Build history of the part. All positions in model axes, mm. Face numbers are marked on the shaded views. A direction names the side the tool comes from. Give positions to 0.01 mm unless a question says otherwise; leave off trailing zeros. Write each loop counter-clockwise with the first axis right and the second up, starting at its lowest first coordinate (ties: lowest second). Pieces come first, ordered by that corner, then holes. Notation, with made-up numbers: (86, 50) -> (92, 50) arc R25 cw to (92, 87) -> close; hole circle Ø10 at (80.25, 7). An arc over 180 degrees is marked (long way). Put each result on its own line as item: value.
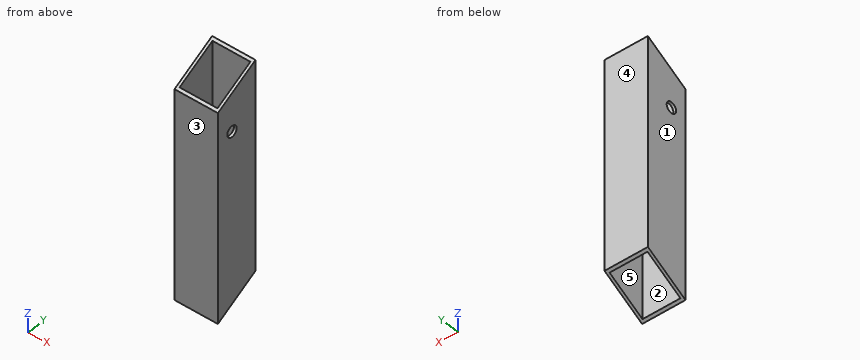
Autodesk Inventor part; units mm, degrees
ref_plane "YZ Plane" through (0, 0, 0) normal (1, 0, 0) x (0, 1, 0)
ref_plane "XZ Plane" through (0, 0, 0) normal (0, 1, 0) x (-1, 0, 0)
ref_plane "XY Plane" through (0, 0, 0) normal (0, 0, 1) x (1, 0, 0)
sketch "Sketch1" plane through (0, 0, 0) normal (0, 0, 1) x (1, 0, 0)
  line L0 (0, 0) -> (25.4, 0)
  line L1 (25.4, 0) -> (25.4, 25.4)
  line L2 (25.4, 25.4) -> (0, 25.4)
  line L3 (0, 25.4) -> (0, 0)
  line L4 (1.5875, 23.8125) -> (23.8125, 23.8125)
  line L5 (23.8125, 23.8125) -> (23.8125, 1.5875)
  line L6 (23.8125, 1.5875) -> (1.5875, 1.5875)
  line L7 (1.5875, 1.5875) -> (1.5875, 23.8125)
  dimension "d0" = 25.4
  dimension "d1" = 25.4
  dimension "d2" = 1.5875
extrude "Extrusion1" add sketch "Sketch1" along normal blind 203.2
sketch "Sketch3" plane through (25.4, 0, 0) normal (1, 0, 0) x (0, 0, -1)
  line L0 (0, 0) -> (-203.2, 0)
  line L1 (0, 0) -> (-14.6647, 25.4)
  line L2 (-14.6647, 25.4) -> (0, 25.4)
  line L3 (0, 23.8125) -> (-203.2, 23.8125)
  line L4 (0, 0) -> (0, 25.4)
  line L5 (0, 25.4) -> (0, 0)
  line L6 (0, 25.4) -> (-203.2, 25.4)
  line L7 (-192.6047, 25.4) -> (-177.94, 0)
  line L8 (0, 25.4) -> (-203.2, 25.4)
  line L9 (-192.6047, 25.4) -> (-203.2, 25.4)
  line L10 (-203.2, 25.4) -> (-203.2, 0)
  line L11 (-177.94, 0) -> (-203.2, 0)
  dimension "d8" = 30
  dimension "d11" = 177.94
extrude "Extrusion3" cut sketch "Sketch3" against normal blind 25.4 contours L1 L3 L4 | L1 L2 L4 L3
sketch "Sketch4" plane through (25.4, 0, 203.2) normal (1, 0, 0) x (0, 0, -1)
  line L0 (14.0789, 25.4) -> (28.7436, 0)
  line L1 (28.7436, 0) -> (0, 0)
  line L2 (189.4518, 23.8125) -> (0, 23.8125)
  line L3 (0, 0) -> (0, 25.4)
  line L4 (0, 25.4) -> (14.0789, 25.4)
  line L5 (188.5353, 25.4) -> (0, 25.4)
  line L6 (203.2, 0) -> (188.5353, 25.4)
  dimension "d12" = 174.4564
  dimension "d13" = 25.4
  dimension "d14" = 28.7436
extrude "Extrusion4" cut sketch "Sketch4" against normal blind 25.4 contours L0 L2 L3 L4 | L0 L1 L3 L2
sketch "Sketch5" plane through (25.4, 0, 174.4564) normal (1, 0, 0) x (0, 0, -1)
  line L0 (173.5398, 1.5875) -> (-0.9165, 1.5875)
  line L1 (173.5398, 1.5875) -> (82.802, -50.8)
  line L2 (174.4564, 0) -> (159.7917, 25.4)
  line L3 (82.802, -50.8) -> (32.002, 37.1882)
  line L4 (159.7917, 25.4) -> (-14.6647, 25.4)
  line L5 (38.8079, 25.4) -> (-14.6647, 25.4)
  line L6 (-14.6647, 25.4) -> (0, 0)
  line L7 (0, 0) -> (53.4726, 0)
  line L8 (-14.6647, 25.4) -> (0, 0)
  line L9 (174.4564, 0) -> (0, 0)
  dimension "d17" = 90
  dimension "d18" = 104.775
  dimension "d20" = 101.6
sketch "Sketch6" plane through (25.4, 0, 174.4564) normal (1, 0, 0) x (0, 0, -1)
  line L0 (159.7917, 25.4) -> (-14.6647, 25.4)
  line L1 (38.8079, 25.4) -> (53.4726, 0)
  line L2 (53.4726, 0) -> (0, 0)
  line L3 (173.5398, 1.5875) -> (-0.9165, 1.5875)
  line L4 (0, 0) -> (-14.6647, 25.4)
  line L5 (0, 0) -> (-14.6647, 25.4)
  line L6 (-14.6647, 25.4) -> (38.8079, 25.4)
  line L7 (160.7082, 23.8125) -> (-13.7482, 23.8125)
  line L8 (174.4564, 0) -> (0, 0)
  line L9 (82.802, -50.8) -> (32.002, 37.1882)
extrude "Extrusion5" cut sketch "Sketch6" against normal blind 25.4
sketch "Sketch7" plane through (25.4, 0, 120.9837) normal (1, 0, 0) x (0, 0, -1)
  line L0 (106.3191, 25.4) -> (-14.6647, 25.4)
  line L1 (-14.6647, 25.4) -> (29.3294, 50.8)
  line L2 (-14.6647, 25.4) -> (0, 0)
  line L3 (16.4978, 9.525) -> (16.4978, 9.525)
  line L4 (16.4978, 9.525) -> (0, 0)
  point P0 (120.9837, 0)
  dimension "d23" = 50.8
  dimension "d25" = 19.05
  dimension "d27" = 0
hole "Hole1" at (25.4, 9.525, 104.486) direction (-1, 0, 0) diameter 6.35 end through all
properties part number "SUP_022_NEWClimberSupport" material "Aluminum 6061"
1) Slice it at D-D (y = 16.75). Write the cut outline in (x, z).
Filled sheet:
outline: (0, 9.67) -> (1.59, 9.67) -> (1.59, 130.65) -> (0, 130.65) -> close; (23.81, 9.67) -> (25.4, 9.67) -> (25.4, 130.65) -> (23.81, 130.65) -> close
2) Tool access for the marked faces 4 and 5: list every direction of +Z, -Z, +X, -X, +Y, -Y with a clear straight run to the whole face (end or side of a thin tool).
Filled sheet:
face 4: +Z, -Z, +X, -X, +Y
face 5: +Z, -Z
3) Wall check: L1, parallel to X at y = 17.5, z = 15; L2, parallel to Y at x = 23.5, z = 129. Give the ranges that are in metal, low to high.
Filled sheet:
L1: 0 to 1.59, 23.81 to 25.4
L2: 23.81 to 25.4
4) Pull direction X, two halves, no side cores. Call the marked faces 1, 2 and 3: released by +X, released by -X, zero draft, split by the parting line, or undercut.
Filled sheet:
face 1: released by -X
face 2: undercut
face 3: zero draft
5) Slice it at A-A (x = 3.5). Write the cut outline in (y, z), plus the area to 3 significant figures.
Filled sheet:
outline: (0, 0) -> (1.59, 0.92) -> (1.59, 121.9) -> (0, 120.98) -> close; (23.81, 13.75) -> (25.4, 14.66) -> (25.4, 135.65) -> (23.81, 134.73) -> close
area: 384 mm2
6) Slice it at B-B (z = 96). Write the cut outline in (x, y).
Filled sheet:
outline: (0, 0) -> (25.4, 0) -> (25.4, 25.4) -> (0, 25.4) -> close; hole (1.59, 1.59) -> (23.81, 1.59) -> (23.81, 23.81) -> (1.59, 23.81) -> close
7) Slice it at C-C (y = 11.5). Write the cut outline in (x, z).
Filled sheet:
outline: (0, 6.64) -> (1.59, 6.64) -> (1.59, 102) -> (0, 102) -> close; (0, 106.97) -> (1.59, 106.97) -> (1.59, 127.62) -> (0, 127.62) -> close; (23.81, 6.64) -> (25.4, 6.64) -> (25.4, 102) -> (23.81, 102) -> close; (23.81, 106.97) -> (25.4, 106.97) -> (25.4, 127.62) -> (23.81, 127.62) -> close
8) Pin check, flat tips, straight feed: pin 1 (3 mm diameter, centred on y = 15, z = 115, fed in from -X); pin 2 (5 mm diameter, centred on y = 9.525, z = 104.486, fed in from +X). Stop position of each tip, or through.
Filled sheet:
pin 1: x = 0
pin 2: through
